```python
from build123d import *

# Parameters (mm, degrees)
F0_R     = 40
F1_DEPTH = 2
F2_R     = 37.2
F2_R_2   = 35
F3_DEPTH = 2
F5_DEPTH = 25
F6_DEPTH = 25


with BuildPart() as f1:
    # F0 (on Front) → F1 (new body)
    with BuildSketch(Plane.XZ):
        Circle(F0_R)
    extrude(amount=F1_DEPTH)

    # F2 (on face) → F3 (join)
    with BuildSketch(Plane.XZ.offset(2)):
        Circle(F2_R)
        Circle(F2_R_2, mode=Mode.SUBTRACT)
    extrude(amount=F3_DEPTH)

    # F4 (on face) → F5 (cut)
    with BuildSketch(Plane.XZ.offset(2)):
        with BuildLine():
            Line((0.6, 7.5), (-0.6, 7.5))
            Line((-0.6, 7.5), (-0.6, 1.374773))
            ThreePointArc((-0.6, 1.374773), (0, 1.5), (0.6, 1.374773))
            Line((0.6, 1.374773), (0.6, 7.5))
        make_face()
        with BuildLine():
            Line((-0.6, 0.75), (-0.6, 1.374773))
            ThreePointArc((-0.6, 1.374773), (-0.999586, 1.118404), (-1.299038, 0.75))
            Line((-1.299038, 0.75), (-0.6, 0.75))
        make_face()
        with BuildLine():
            ThreePointArc((1.299038, 0.75), (0.999586, 1.118404), (0.6, 1.374773))
            Line((0.6, 1.374773), (0.6, 0.75))
            Line((0.6, 0.75), (1.299038, 0.75))
        make_face()
        with BuildLine():
            ThreePointArc((-1.299038, -0.75), (-1.5, 0), (-1.299038, 0.75))
            Line((-1.299038, 0.75), (-7.5, 0.75))
            Line((-7.5, 0.75), (-7.5, -0.75))
            Line((-7.5, -0.75), (-1.299038, -0.75))
        make_face()
        with BuildLine():
            Line((7.5, 0.75), (1.299038, 0.75))
            ThreePointArc((1.299038, 0.75), (1.448889, 0.388229), (1.5, 0))
            ThreePointArc((1.5, 0), (1.448889, -0.388229), (1.299038, -0.75))
            Line((1.299038, -0.75), (7.5, -0.75))
            Line((7.5, -0.75), (7.5, 0.75))
        make_face()
        with BuildLine():
            Line((-0.6, -1.374773), (-0.6, -0.75))
            Line((-0.6, -0.75), (-1.299038, -0.75))
            ThreePointArc((-1.299038, -0.75), (-0.999586, -1.118404), (-0.6, -1.374773))
        make_face()
        with BuildLine():
            Line((1.299038, -0.75), (0.6, -0.75))
            Line((0.6, -0.75), (0.6, -1.374773))
            ThreePointArc((0.6, -1.374773), (0.999586, -1.118404), (1.299038, -0.75))
        make_face()
        with BuildLine():
            ThreePointArc((0.6, -1.374773), (0, -1.5), (-0.6, -1.374773))
            Line((-0.6, -1.374773), (-0.6, -7.5))
            Line((-0.6, -7.5), (0.6, -7.5))
            Line((0.6, -7.5), (0.6, -1.374773))
        make_face()
    extrude(amount=-F5_DEPTH, mode=Mode.SUBTRACT)

    # F5_face (on face) → F6 (cut)
    with BuildSketch(Plane.XZ.offset(2)):
        with BuildLine():
            ThreePointArc((-0.6, -1.374773), (0, -1.5), (0.6, -1.374773))
            Line((0.6, -1.374773), (0.6, -0.75))
            Line((0.6, -0.75), (1.299038, -0.75))
            ThreePointArc((1.299038, -0.75), (1.5, 0), (1.299038, 0.75))
            Line((1.299038, 0.75), (0.6, 0.75))
            Line((0.6, 0.75), (0.6, 1.374773))
            ThreePointArc((0.6, 1.374773), (0, 1.5), (-0.6, 1.374773))
            Line((-0.6, 1.374773), (-0.6, 0.75))
            Line((-0.6, 0.75), (-1.299038, 0.75))
            ThreePointArc((-1.299038, 0.75), (-1.5, 0), (-1.299038, -0.75))
            Line((-1.299038, -0.75), (-0.6, -0.75))
            Line((-0.6, -0.75), (-0.6, -1.374773))
        make_face()
    extrude(amount=-F6_DEPTH, mode=Mode.SUBTRACT)


solid = f1.part
```
The listing builds one solid part. Answer for the finished solid, in the listing's coordinates (mm). A direction names the side the tool comes from. Give positions to 0.01 mm unless a question says otherwise; leave off trailing zeros. Order: outer loops, then holes, each group sorted by start corner. A loop starts at its lowest first (then second) coordinate and runs counter-clockwise, first axis right, second up. Notation, with made-up numbers: (87.25, 84.25) - (98.25, 84.25) arc R30 ccw to (98.25, 114.25) - close; hole circle Ø3 at (78, 21.5). An arc over 180 degrees is marked (long way). Use one line per item in the form item = value. Start each with the question number.
(1) Consider line 1 (Z direction, x = 0, y = -3.15); line 2 (Y direction, x = 31, z = 15.5); line 3 (Z direction, x = -5.5, y = -2.4). Determine where each line is inside the solid, lowest interval first. Write a range as from..to.
(2) The mould has two halves that part along Z. Classify faces 1 (the flat face through (-0.6, -1, -4)), 2 (the flat face through (8, 0, 1)), 3 (the flat face through (0.6, -1, 4)), 4 (the cylindrical face through (-8.67, -0.99, -39.05)): released by +Z, released by -Z, zero draft, split by the parting line, or undercut.
(3) For faces 5 (the flat face through (-8, -2, 0)), 6 (the flat face through (0.6, -1, -4)), 7 (the flat face through (-25, -4, -25)), determine the directions among +Z, -Z, +X, -X, +Y, -Y from which every point of the face is accessible in a straight line to the end or side of a thin tool.
(4) A cutting plane is placed at B-B, the plane x = 16.5. Write down the section's boundary in (y, z).
(5) A cutting plane is placed at C-C, the plane z = -34. Write down the section's boundary in (x, y), then the cut area to 3 significant figures.
(6) Flat-ended cylindrical pins translate along their axes: pin 1 Ø10 at (x, z) = (1.5, 12) entering from -Y; pin 2 Ø0.6 at (y, z) = (-1, -3.5) entering from +X; pin 3 Ø1 at (y, z) = (-1, 4) entering from -X. Find the tip coordinate at first contact, or state that the pin passes through.
(7) A cutting plane is placed at A-A, the plane y = -3.05. Write down the section's boundary in (x, z), then the cut area to 3 significant figures.
Ans:
q1.line_1 = -37.2..-35, 35..37.2
q1.line_2 = -2..0
q1.line_3 = -36.79..-34.57, 34.57..36.79
q2.face_1 = undercut
q2.face_2 = zero draft
q2.face_3 = undercut
q2.face_4 = split by the parting line
q3.face_5 = -Y
q3.face_6 = +Y, -Y
q3.face_7 = +Z, -Z, +X, -X, -Y
q4.outline = (-4, -33.34) - (-2, -33.34) - (-2, -36.44) - (0, -36.44) - (0, 36.44) - (-2, 36.44) - (-2, 33.34) - (-4, 33.34) - (-4, 30.87) - (-2, 30.87) - (-2, -30.87) - (-4, -30.87) - close
q5.outline = (-21.07, -2) - (-15.09, -2) - (-15.09, -4) - (-8.31, -4) - (-8.31, -2) - (8.31, -2) - (8.31, -4) - (15.09, -4) - (15.09, -2) - (21.07, -2) - (21.07, 0) - (-21.07, 0) - close
q5.area = 111 mm^2
q6.pin_1 = -2
q6.pin_2 = 39.87
q6.pin_3 = -39.85
q7.outline = circle Ø74.4 at (0, 0); hole circle Ø70 at (0, 0)
q7.area = 499 mm^2
